```python
from build123d import *

# Parameters (mm, degrees)
SKETCH1_W                 = 76.2
SKETCH1_H                 = 107.95
BOSS_EXTRUDE1_DEPTH       = 6.35
SKETCH2_R                 = 1.7526
SKETCH2_W                 = 12.7
SKETCH2_H                 = 6.35
SKETCH2_W_2               = 25.4
CUT_EXTRUDE1_DEPTH        = 6.35
CUT_EXTRUDE2_REACH        = 68.372
SKETCH3_W                 = 25.4
SKETCH3_H                 = 38.1
F_6_CLEARANCE_HOLE1_D     = 3.5052
F_6_CLEARANCE_HOLE1_DEPTH = 6.35
F_6_CLEARANCE_HOLE1_TIP   = 1.053068321
F_1_4_CLEARANCE_HOLE1_D   = 6.7564


with BuildPart() as part:
    # Sketch1 → Boss-Extrude1 (new body)
    with BuildSketch(Plane(origin=(0, 0, 0), x_dir=(1, 0, 0), z_dir=(0, 1, 0))):
        Rectangle(SKETCH1_W, SKETCH1_H)
    extrude(amount=BOSS_EXTRUDE1_DEPTH)

    # Sketch2 → Cut-Extrude1 (cut)
    with BuildSketch(Plane(origin=(0, 6.35, 0), x_dir=(1, 0, 0), z_dir=(0, 1, 0))):
        with Locations(Location((-19.05, 50.8, 0), (0, 0, 270))):
            Circle(SKETCH2_R)
        with Locations(Location((19.05, 50.8, 0), (0, 0, 270))):
            Circle(SKETCH2_R)
        with Locations(Location((19.05, -50.8, 0), (0, 0, 90))):
            Circle(SKETCH2_R)
        with Locations(Location((-19.05, -50.8, 0), (0, 0, 90))):
            Circle(SKETCH2_R)
        with Locations((-31.75, 50.8)):
            Rectangle(SKETCH2_W, SKETCH2_H)
        with Locations((0, 50.8)):
            Rectangle(SKETCH2_W_2, SKETCH2_H)
        with Locations((31.75, 50.8)):
            Rectangle(SKETCH2_W, SKETCH2_H)
        with Locations((31.75, -50.8)):
            Rectangle(SKETCH2_W, SKETCH2_H)
        with Locations((0, -50.8)):
            Rectangle(SKETCH2_W_2, SKETCH2_H)
        with Locations((-31.75, -50.8)):
            Rectangle(SKETCH2_W, SKETCH2_H)
    extrude(amount=-CUT_EXTRUDE1_DEPTH, mode=Mode.SUBTRACT)

    # Sketch3 → Cut-Extrude2 (cut, up to next)
    with BuildSketch(Plane(origin=(0, 6.35, 0), x_dir=(1, 0, 0), z_dir=(0, 1, 0)), mode=Mode.PRIVATE) as cut_extrude2_sk1:
        with Locations((25.4, 0)):
            Rectangle(SKETCH3_W, SKETCH3_H)
    cut_extrude2_tool1 = extrude(cut_extrude2_sk1.sketch, amount=-CUT_EXTRUDE2_REACH, mode=Mode.PRIVATE) & part.part
    add(cut_extrude2_tool1.solids().sort_by_distance((25.4, 6.35, 0))[0], mode=Mode.SUBTRACT)

    # #6 Clearance Hole1
    with Locations(Plane(origin=(0, 6.35, 0), x_dir=(1, 0, 0), z_dir=(0, 1, 0))):
        with Locations((-19.05, 50.8), (19.05, 50.8), (-19.05, -50.8), (19.05, -50.8)):
            Hole(F_6_CLEARANCE_HOLE1_D / 2, depth=F_6_CLEARANCE_HOLE1_DEPTH)
            with Locations((0, 0, -(F_6_CLEARANCE_HOLE1_DEPTH + F_6_CLEARANCE_HOLE1_TIP / 2))):  # 118° drill point
                Cone(0, F_6_CLEARANCE_HOLE1_D / 2, F_6_CLEARANCE_HOLE1_TIP, mode=Mode.SUBTRACT)

    # 1/4 Clearance Hole1 (through all)
    with Locations(Plane(origin=(0, 0, 0), x_dir=(-1, 0, 0), z_dir=(0, -1, 0))):
        with Locations((-25.4, 31.75), (-25.4, -31.75)):
            Hole(F_1_4_CLEARANCE_HOLE1_D / 2)


solid = part.part
```
Check sheet for the modelled part. Datum: model origin and axes. Units: mm. A direction names the side the tool comes from. Give positions to 0.01 mm unless a question says otherwise; leave off trailing zeros. Order: outer loops, then holes, each group sorted by start corner. A loop starts at its lowest first (then second) coordinate and runs counter-clockwise, first axis right, second up. Notation, with made-up numbers: M 76,-31 L 130,-31 A18 cw 130,-27 Z; hole C 58,82 d3. An arc over 180 degrees is marked long. Answer in a Markdown table with one row per item. Add a question column.
Q1. Sectioned sample at B-B, the plane y = 2.5. Count the separate pieces of the cut face and the enclosed holes in it, and give its area (3 significant figures).
Q2. Gauge pin test, flat ends, axial feed: pin 1 Ø1.9 at (x, y) = (-31.5, 2.5) entering from +Z (3 decimals); pin 2 Ø4 at (x, z) = (19.05, 50.8) entering from -Y; pin 3 Ø1.9 at (y, z) = (4.5, 50.5) entering from +X; pin 4 Ø1 at (x, y) = (11.5, 5.5) entering from -Z (3 decimals). Record the tip position at first contact, or that the pin passes through.
Q3. Sectioned sample at D-D, the plane z = -31.75. Record the boundary of the cut face in (x, y), and give its area (3 significant figures).
Q4. Release check for a two-part mould opening along Z. For faces 6 (the flat face through (25.4, 3, 51)), 7 (the flat face through (32, 3, 47.625)), 8 (the flat face through (19, 3, -53.975)), 9 (the flat face through (12.7, 3, 0)) record: released by +Z, released by -Z, zero draft, split by the parting line, or undercut.
Q5. Thickness scan on L1, parallel to X at y = 2.5, z = 50.8; L2, parallel to Z at x = -18, y = 4.5 (3 decimals); L3, parallel to X at y = 1.75, z = 31.75. Record the ranges inside material, lowest first.
Q6. Access from +Z, -Z, +X, -X, +Y, -Y to the whole of each face (thin tool, end or side, straight path). Record for faces 1 (the flat face through (-12.7, 3, -51)), 2 (the flat face through (25.4, 3, -51)), 3 (the flat face through (0, 3, 47.625)), 4 (the flat face through (-32, 3, -47.625)), 5 (the flat face through (25, 3, -19.05)).
Q7. Sectioned sample at A-A, the plane x = 19.05. Record the boundary of the cut face in (y, z) (3 decimals), and give its area (3 significant figures).
Q8. Sectioned sample at C-C, the plane x = -19.05. Record the boundary of the cut face in (y, z) (3 decimals).
Verdict:
| question | item | result |
|---|---|---|
| 1 | separate pieces | 1 |
| 1 | enclosed holes | 6 |
| 1 | area | 6,500 mm² |
| 2 | pin 1 | z = 47.625 |
| 2 | pin 2 | y = 0 |
| 2 | pin 3 | x = 25.4 |
| 2 | pin 4 | z = -47.625 |
| 3 | outline | M -38.1,0 L 22.02,0 L 22.02,6.35 L -38.1,6.35 Z; M 28.78,0 L 38.1,0 L 38.1,6.35 L 28.78,6.35 Z |
| 3 | area | 441 mm² |
| 4 | face 6 | zero draft |
| 4 | face 7 | released by +Z |
| 4 | face 8 | released by -Z |
| 4 | face 9 | undercut |
| 5 | L1 | -25.4 to -20.8, -17.3 to -12.7, 12.7 to 17.3, 20.8 to 25.4 |
| 5 | L2 | -53.975 to -52.203, -49.397 to 49.397, 52.203 to 53.975 |
| 5 | L3 | -38.1 to 22.02, 28.78 to 38.1 |
| 6 | face 1 | -Z, +Y, -Y |
| 6 | face 2 | -Z, +X, +Y, -Y |
| 6 | face 3 | +Z, +Y, -Y |
| 6 | face 4 | -Z, -X, +Y, -Y |
| 6 | face 5 | +X, +Y, -Y |
| 7 | outline | M 0,-53.975 L 6.35,-53.975 L 6.35,-52.553 L 0,-52.553 Z; M 0,-49.047 L 6.35,-49.047 L 6.35,-19.05 L 0,-19.05 Z; M 0,19.05 L 6.35,19.05 L 6.35,49.047 L 0,49.047 Z; M 0,52.553 L 6.35,52.553 L 6.35,53.975 L 0,53.975 Z |
| 7 | area | 399 mm² |
| 8 | outline | M 0,-53.975 L 6.35,-53.975 L 6.35,-52.553 L 0,-52.553 Z; M 0,-49.047 L 6.35,-49.047 L 6.35,49.047 L 0,49.047 Z; M 0,52.553 L 6.35,52.553 L 6.35,53.975 L 0,53.975 Z |
